For this review, take the finished solid that the model builds, in its own axes (mm). Round coordinates to 2 decimals unless told otherwise and drop trailing zeros. Order: outer loops, then holes, each group sorted by start corner. A loop starts at its lowest first (then second) coordinate and runs counter-clockwise, first axis right, second up. Notation, with made-up numbers: M 86.25,68.5 L 111.25,68.5 A10 cw 111.25,73.5 Z; hole C 27.25,10.5 d6. An arc over 180 degrees is marked long. Put each result on its own line as item: value.
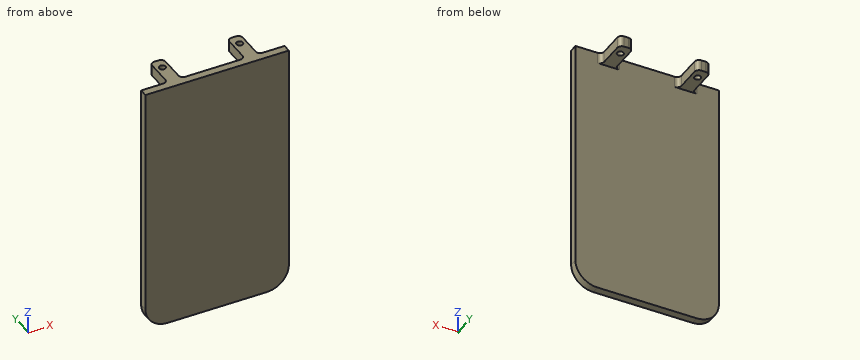
from build123d import *

# Parameters (mm, degrees)
SKETCH_1_W      = 65
SKETCH_1_H      = 115
EXTRUDE_1_DEPTH = 3.6
SKETCH_3_W      = 6
SKETCH_3_H      = 15
SKETCH_3_R      = 1.45
EXTRUDE_2_DEPTH = 5
FILLET_1_R      = 10
FILLET_2_R      = 2


with BuildPart() as part:
    # 草图1 → 凸台-拉伸1 (new body)
    with BuildSketch(Plane(origin=(0, 0, 0), x_dir=(1, 0, 0), z_dir=(0, 1, 0))):
        with Locations((-5.550310529, -31.459318732)):
            Rectangle(SKETCH_1_W, SKETCH_1_H)
    extrude(amount=EXTRUDE_1_DEPTH)

    # 草图3 → 凸台-拉伸2 (add)
    with BuildSketch(Plane.XY.offset(88.959318732)):
        with Locations((-23.050310529, 11.1)):
            Rectangle(SKETCH_3_W, SKETCH_3_H)
        with Locations((-23.050310529, 13.6)):
            Circle(SKETCH_3_R, mode=Mode.SUBTRACT)
        with Locations((11.949689471, 11.1)):
            Rectangle(SKETCH_3_W, SKETCH_3_H)
        with Locations((11.949689471, 13.6)):
            Circle(SKETCH_3_R, mode=Mode.SUBTRACT)
    extrude(amount=-EXTRUDE_2_DEPTH)

    # 圆角1
    fillet_1_edges = [part.edges().sort_by_distance(p)[0] for p in [
        (-38.050310529, 1.8, -26.040681268),
        (26.949689471, 1.8, -26.040681268),
    ]]
    fillet(fillet_1_edges, radius=FILLET_1_R)

    # 圆角2
    fillet_2_edges = [part.edges().sort_by_distance(p)[0] for p in [
        (-26.050310529, 3.6, 86.459318732),
        (-26.050310529, 18.6, 86.459318732),
        (-20.050310529, 18.6, 86.459318732),
        (-20.050310529, 3.6, 86.459318732),
        (14.949689471, 18.6, 86.459318732),
        (14.949689471, 3.6, 86.459318732),
        (8.949689471, 3.6, 86.459318732),
        (8.949689471, 18.6, 86.459318732),
    ]]
    fillet(fillet_2_edges, radius=FILLET_2_R)


solid = part.part
(1) Insertion check: pin 1 Ø3.5 at (x, y) = (11.95, 13.6) entering from -Z; pin 2 Ø1.5 at (y, z) = (12.5, 87.5) entering from -X; pin 3 Ø2.5 at (y, z) = (9, 87) entering from +X. Each pin has a flat end and moves straight along its axis. Give the tip position at first contact, or say it passes through.
A:
pin 1: stops at z = 83.96
pin 2: stops at x = -26.05
pin 3: stops at x = 14.95
(2) To check wall thickness, follow L1, parallel to Y at x = -2.5, z = -18; L2, parallel to Z at x = -26, y = 6.5; L3, parallel to Z at x = -34, y = 1.5. State the ranges of each line that lie inside material, in increasing order.
A:
L1: y = 0 to 3.6
L2: z = 83.96 to 88.96
L3: z = -24.08 to 88.96
(3) Add section B-B on y = 13.6. Give the boundary of the cut face in (x, z).
A:
outline: M -26.05,83.96 L -24.5,83.96 L -24.5,88.96 L -26.05,88.96 Z; M -21.6,83.96 L -20.05,83.96 L -20.05,88.96 L -21.6,88.96 Z; M 8.95,83.96 L 10.5,83.96 L 10.5,88.96 L 8.95,88.96 Z; M 13.4,83.96 L 14.95,83.96 L 14.95,88.96 L 13.4,88.96 Z
(4) Add section A-A on y = 7.5. Give the boundary of the cut face in (x, z).
A:
outline: M -26.05,83.96 L -20.05,83.96 L -20.05,88.96 L -26.05,88.96 Z; M 8.95,83.96 L 14.95,83.96 L 14.95,88.96 L 8.95,88.96 Z
(5) Add section D-D on x = 20. Give the boundary of the cut face in (y, z).
A:
outline: M 0,-25.56 L 3.6,-25.56 L 3.6,88.96 L 0,88.96 Z
(6) Add section C-C on z = 75. Give the boundary of the cut face in (x, y).
A:
outline: M -38.05,0 L 26.95,0 L 26.95,3.6 L -38.05,3.6 Z
